```python
from build123d import *

# Parameters (mm, degrees)
SKETCH1_W           = 40.64
SKETCH1_H           = 19.05
SKETCH1_R           = 3.302
SKETCH1_H_2         = 38.735
SKETCH1_R_2         = 1.9812
SKETCH1_R_3         = 11.049
BOSS_EXTRUDE1_DEPTH = 5.08


with BuildPart() as part:
    # Sketch1 → Boss-Extrude1 (new body)
    with BuildSketch(Plane.XY):
        with Locations((5.46838271, -19.760168498)):
            Rectangle(SKETCH1_W, SKETCH1_H)
        with Locations((-7.23161729, -19.760168498)):
            Circle(SKETCH1_R, mode=Mode.SUBTRACT)
        with Locations((18.16838271, -19.760168498)):
            Circle(SKETCH1_R, mode=Mode.SUBTRACT)
        with Locations((5.46838271, 9.132331502)):
            Rectangle(SKETCH1_W, SKETCH1_H_2)
        with Locations((-7.494416142, -2.225366655)):
            Circle(SKETCH1_R_2, mode=Mode.SUBTRACT)
        with Locations((18.413583858, -2.242964365)):
            Circle(SKETCH1_R_2, mode=Mode.SUBTRACT)
        with Locations((-7.476818437, 23.682627368)):
            Circle(SKETCH1_R_2, mode=Mode.SUBTRACT)
        with Locations((5.46838271, 10.719831502)):
            Circle(SKETCH1_R_3, mode=Mode.SUBTRACT)
        with Locations((18.431181563, 23.665029659)):
            Circle(SKETCH1_R_2, mode=Mode.SUBTRACT)
    extrude(amount=BOSS_EXTRUDE1_DEPTH)


solid = part.part
```
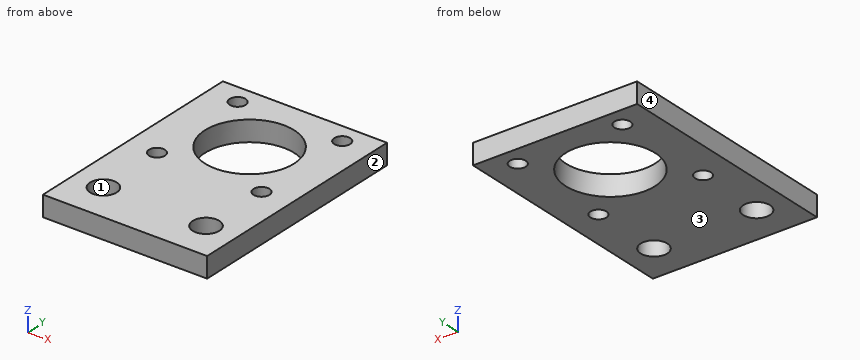
Build history of the part. All positions in model axes, mm. Face numbers are marked on the shaded views. Round coordinates to 2 decimals unless told otherwise and drop trailing zeros. Write each loop counter-clockwise with the first axis right and the second up, starting at its lowest first coordinate (ties: lowest second). Pieces come first, ordered by that corner, then holes. Notation, with made-up numbers: (56.5, 47.5) -> (115.5, 47.5) arc R35 ccw to (115.5, 80.5) -> close; hole circle Ø11 at (-14.75, 45). An arc over 180 degrees is marked (long way). Put each result on its own line as item: value.
Item 1: Two-plate mould, pull along X, no slides. Class the marked faces 1, 2, 3 and 4: pulls with the +X half, pulls with the -X half, needs draft (parallel to the pull), parting line crosses it, or undercut.
Here are the results:
face 1: undercut
face 2: pulls with the +X half
face 3: needs draft
face 4: pulls with the -X half
Item 2: Flat gauge pins, fed straight in: P1, Ø1.5, axis at x = 19, y = -22, coming from the +Z side; P2, Ø6.5, axis at x = 18.41, y = -2.24, coming from the +Z side. Where does each tip first touch, or does it go through?
Here are the results:
P1: passes through
P2: stops at z = 5.08
Item 3: Slice it at C-C, the plane y = 18. Give the cut face in (x, z).
Here are the results:
outline: (-14.85, 0) -> (-2.84, 0) -> (-2.84, 5.08) -> (-14.85, 5.08) -> close; (13.78, 0) -> (25.79, 0) -> (25.79, 5.08) -> (13.78, 5.08) -> close
Item 4: Slice it at A-A, the plane x = 10.5. Give the cut face in (y, z), plus the area to 3 significant figures.
Here are the results:
outline: (-29.29, 0) -> (0.88, 0) -> (0.88, 5.08) -> (-29.29, 5.08) -> close; (20.56, 0) -> (28.5, 0) -> (28.5, 5.08) -> (20.56, 5.08) -> close
area: 194 mm^2
Item 5: Slice it at B-B, the plane z = 3.95. Give the cut face in (x, y).
Here are the results:
outline: (-14.85, -29.29) -> (25.79, -29.29) -> (25.79, 28.5) -> (-14.85, 28.5) -> close; hole circle Ø6.6 at (-7.23, -19.76); hole circle Ø3.96 at (-7.49, -2.23); hole circle Ø3.96 at (-7.48, 23.68); hole circle Ø22.1 at (5.47, 10.72); hole circle Ø6.6 at (18.17, -19.76); hole circle Ø3.96 at (18.41, -2.24); hole circle Ø3.96 at (18.43, 23.67)
Item 6: Wall check: probe 1 along X at (y, z) = (-19, 4.3); probe 2 along X at (y, z) = (-18.5, 1.75); probe 3 along Y at (x, z) = (-6, 3). Give the ranges that are in metal, low to high. Write a range as from..to.
Here are the results:
probe 1: x = -14.85..-10.44, -4.02..14.96, 21.38..25.79
probe 2: x = -14.85..-10.28, -4.18..15.12, 21.22..25.79
probe 3: y = -29.29..-22.82, -16.7..-3.53, -0.92..22.36, 25..28.5
